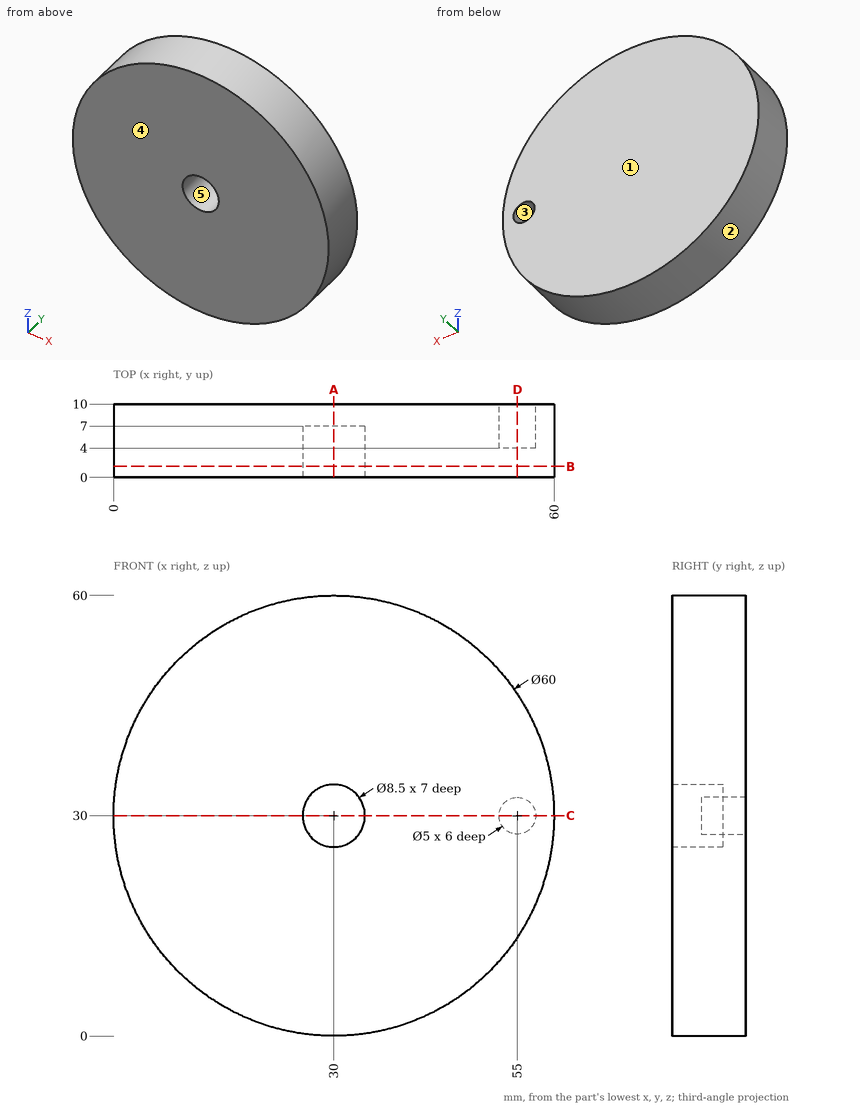
Input: dimensioned drawing with shaded views. Units: mm. Origin: part minimum x, y, z. A direction names the side the tool comes from. Give positions to 0.01 mm unless a question says otherwise; leave off trailing zeros. Write each loop counter-clockwise with the first axis right and the second up, starting at its lowest first coordinate (ties: lowest second). Pieces come first, ordered by that corner, then holes. Notation, with made-up numbers: (83, 29) -> (114, 29) arc R16 cw to (114, 46) -> close; hole circle Ø5 at (-6, -4). An arc over 180 degrees is marked (long way). Return JSON: item names as keys, results as strings. Group by question number.
1. Section D-D, the plane x = 55. Output: boundary loops of the cut face in (y, z).
2. Section C-C, the plane z = 30. Output: boundary loops of the cut face in (x, y).
3. Mould query, pull axis Z, two halves, no side actions, for the marked faces 1, 2 and 3. Classes: +Z half, -Z half, draft (parallel to the pull), parting line (faces both ways), or undercut.
4. Section A-A, the plane x = 30. Output: boundary loops of the cut face in (y, z), then the cut area to 4 significant figures.
5. Pin query (flat end, axial travel): pin 1 Ø2 at (y, z) = (3, 41) entering from -X; pin 2 Ø4 at (x, y) = (46.5, 4.5) entering from -Z; pin 3 Ø1.5 at (x, y) = (36, 1.5) entering from +Z. Return the tip coordinate at first contact, or that it passes through.
6. Access query for the marked faces 4 and 5. Directions: +Z, -Z, +X, -X, +Y, -Y. A direction counts if a zero-diameter tool reaches every point of the face in a straight line with its end or side. Return the directions, or none.
7. Section B-B, the plane y = 1.5. Output: boundary loops of the cut face in (x, z).
8. Material intervals for line 1 (X direction, y = 5.6, z = 30); line 2 (X direction, y = 7.3, z = 30); line 3 (X direction, y = 4.75, z = 28), sorted ascending. Write a range as from..to.
Determined:
{
 "1": {"outline": "(0, 13.42) -> (10, 13.42) -> (10, 27.5) -> (4, 27.5) -> (4, 32.5) -> (10, 32.5) -> (10, 46.58) -> (0, 46.58) -> close"},
 "2": {"outline": "(0, 0) -> (25.75, 0) -> (25.75, 7) -> (34.25, 7) -> (34.25, 0) -> (60, 0) -> (60, 10) -> (57.5, 10) -> (57.5, 4) -> (52.5, 4) -> (52.5, 10) -> (0, 10) -> close"},
 "3": {"face 1": "draft", "face 2": "parting line", "face 3": "undercut"},
 "4": {"outline": "(0, 0) -> (10, 0) -> (10, 60) -> (0, 60) -> (0, 34.25) -> (7, 34.25) -> (7, 25.75) -> (0, 25.75) -> close", "area": "540.5 mm2"},
 "5": {"pin 1": "stops at x = 1.72", "pin 2": "stops at z = 3.74", "pin 3": "stops at z = 59.54"},
 "6": {"face 4": "+Z, -Z, +X, -X, -Y", "face 5": "-Y"},
 "7": {"outline": "circle Ø60 at (30, 30); hole circle Ø8.5 at (30, 30)"},
 "8": {"line 1": "x = 0..25.75, 34.25..52.5, 57.5..60", "line 2": "x = 0..52.5, 57.5..60", "line 3": "x = 0.07..26.25, 33.75..53.5, 56.5..59.93"}
}
